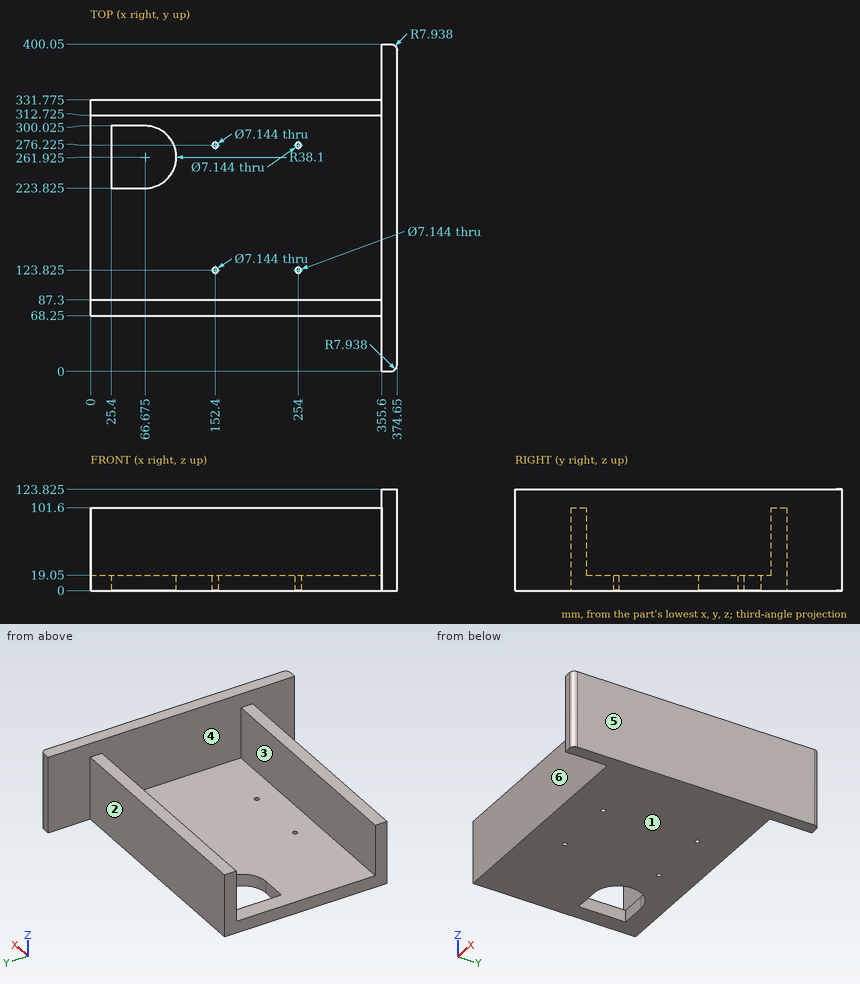
Input: dimensioned drawing with shaded views. Units: mm. Origin: part minimum x, y, z. A direction names the side the tool comes from. Coordinates: 2 decimals unless noted, no trailing zeros. Write each question's results on one line, items separated by ' | '. Start each with the question number.
Item 1: First-contact query: pin 1 Ø10 at (y, z) = (299, 27.5) entering from -X; pin 2 Ø6 at (x, y) = (310.5, 77.5) entering from +Z; pin 3 Ø21 at (x, z) = (51.5, 6.5) entering from -Y; pin 4 Ø5.5 at (x, y) = (254, 276.225) entering from -Z. Flat tips, straight axial feed; report the tip coordinate or a pass-through.
Item 2: Draft query along Y for the marked faces 4, 5 and 6. Return one class per face: pulls with the +Y half, pulls with the -Y half, needs draft (parallel to the pull), parting line crosses it, or undercut.
Item 3: Set-up query: the marked faces 1, 2 and 3. Return all of +Z, -Z, +X, -X, +Y, -Y with unobstructed straight access to the full face (end or side cutting, diameter ignored); none if empty.
Item 4: Line query: probe 1 along Z at (x, y) = (103.5, 189.5); probe 2 along X at (y, z) = (110.5, 117.5); probe 3 along Z at (x, y) = (272, 323.5). Output: solid intervals per line, ascending.
Checked values:
1) pin 1: stops at x = 355.6 | pin 2: stops at z = 101.6 | pin 3: stops at y = 68.25 | pin 4: passes through
2) face 4: undercut | face 5: needs draft | face 6: pulls with the -Y half
3) face 1: -Z, +X, -X, +Y, -Y | face 2: +Z, -Z, -X, +Y | face 3: +Z, -X
4) probe 1: z = 0 to 19.05 | probe 2: x = 355.6 to 374.65 | probe 3: z = 0 to 101.6
